from build123d import *

# Parameters (mm, degrees)
F0_W     = 61.4049248397
F0_H     = 137.3135596514
F1_DEPTH = 228.6
F2_T     = -2.54
F7_R     = 5.08


# Not quite as in the source:
# - the program builds the solid bodies; features that only make, move or delete a surface that nothing else refers to are left out


with BuildPart() as f1:
    # F0 (on Top) → F1 (new body)
    with BuildSketch(Plane.XY):
        with Locations((30.7024624199, 68.6567798257)):
            Rectangle(F0_W, F0_H)
    extrude(amount=F1_DEPTH)

    # F2
    f2_openings = [f1.faces().sort_by_distance(p)[0] for p in [
        (0, 68.65678, 114.3),
    ]]
    offset(amount=F2_T, openings=f2_openings)

    # F7
    f7_edges = [f1.edges().sort_by_distance(p)[0] for p in [
        (58.864925, 134.77356, 114.3),
        (58.864925, 68.65678, 2.54),
        (58.864925, 2.54, 114.3),
        (58.864925, 68.65678, 226.06),
    ]]
    fillet(f7_edges, radius=F7_R)


solid = f1.part
Check sheet for the modelled part. Datum: model origin and axes. Units: mm. A direction names the side the tool comes from. Coordinates: 2 decimals unless noted, no trailing zeros. Write each loop counter-clockwise with the first axis right and the second up, starting at its lowest first coordinate (ties: lowest second). Pieces come first, ordered by that corner, then holes.
Item 1: Cross-section at A-A on x = 17.5. Record the boundary of the cut face in (y, z), then the cut area to 3 significant figures.
Numbers:
outline: (0, 0) - (137.31, 0) - (137.31, 228.6) - (0, 228.6) - close; hole (2.54, 2.54) - (134.77, 2.54) - (134.77, 226.06) - (2.54, 226.06) - close
area: 1,830 mm2
Item 2: Cross-section at C-C on z = 174. Record the boundary of the cut face in (x, y).
Numbers:
outline: (0, 0) - (61.4, 0) - (61.4, 137.31) - (0, 137.31) - (0, 134.77) - (53.78, 134.77) arc R5.08 cw to (58.86, 129.69) - (58.86, 7.62) arc R5.08 cw to (53.78, 2.54) - (0, 2.54) - close
Item 3: Scan lines: probe 1 along Z at (x, y) = (18.5, 6.5); probe 2 along Y at (x, z) = (10.5, 184); probe 3 along X at (y, z) = (72, 159). Record each from-to range of solid material in increasing order.
Numbers:
probe 1: z = 0 to 2.54, 226.06 to 228.6
probe 2: y = 0 to 2.54, 134.77 to 137.31
probe 3: x = 58.86 to 61.4
Item 4: Depth check by flat-ended pin: pin 1 Ø1 at (y, z) = (36.5, 72.5) entering from -X. Enter the tip coordinate at first touch or a pass-through.
Numbers:
pin 1: stops at x = 58.86
Item 5: Access from +Z, -Z, +X, -X, +Y, -Y to the whole of each face (thin tool, end or side, straight path). Record for faces 1 (the face through (61.405, 68, 113)), 2 (the face through (57.34, 3.99, 115.86)).
Numbers:
face 1: +Z, -Z, +X, +Y, -Y
face 2: -X
Item 6: Cross-section at B-B on y = 35. Record the boundary of the cut face in (x, z), then the cut area to 3 significant figures.
Numbers:
outline: (0, 0) - (61.4, 0) - (61.4, 228.6) - (0, 228.6) - (0, 226.06) - (53.78, 226.06) arc R5.08 cw to (58.86, 220.98) - (58.86, 7.62) arc R5.08 cw to (53.78, 2.54) - (0, 2.54) - close
area: 891 mm2
Item 7: Mould release check, pull along Z, two halves, no side actions. Record for faces 3 (the face through (30, 70, 228.6)), 4 (the face through (58.865, 68, 113)), 5 (the face through (30, 0, 113)), 6 (the face through (27, 70, 2.54)): released by +Z, released by -Z, zero draft, split by the parting line, or undercut.
Numbers:
face 3: released by +Z
face 4: undercut
face 5: zero draft
face 6: undercut
